Can you work these out from the model? Positions are in its coordinate system, mm. Coordinates: 2 decimals unless noted, no trailing zeros. Order: outer loops, then holes, each group sorted by start corner. A loop starts at its lowest first (then second) coordinate and runs counter-clockwise, first axis right, second up.
Autodesk Inventor part; units mm, degrees
ref_plane "Start Plane" through (0, 0, -57.0711) normal (0, 0, 1) x (1, 0, 0)
ref_plane "End Plane" through (0, 0, 2457.0711) normal (0, 0, 1) x (1, 0, 0)
ref_plane "Work Plane4" through (-60, 0, 2460) normal (0.7071, 0, 0.7071) x (0.7071, 0, -0.7071)
ref_plane "Start Plane" through (0, 0, -57.0711) normal (0, 0, 1) x (1, 0, 0)
ref_plane "End Plane" through (0, 0, 2457.0711) normal (0, 0, 1) x (1, 0, 0)
sketch "Sketch" plane through (0, 0, 0) normal (0, 0, 1) x (1, 0, 0)
  line L0 (-60, -50) -> (-60, 50)
  line L1 (-50, 60) -> (50, 60)
  line L2 (60, 50) -> (60, -50)
  line L3 (50, -60) -> (-50, -60)
  arc A0 (-60, -50) -> (-50, -60) centre (-50, -50) ccw
  arc A1 (60, 50) -> (50, 60) centre (50, 50) ccw
  arc A2 (-50, 60) -> (-60, 50) centre (-50, 50) ccw
  arc A3 (50, -60) -> (60, -50) centre (50, -50) ccw
  arc A4 (-50, 55) -> (-55, 50) centre (-50, 50) ccw
  line L4 (-50, 55) -> (50, 55)
  arc A5 (55, 50) -> (50, 55) centre (50, 50) ccw
  line L5 (55, 50) -> (55, -50)
  arc A6 (50, -55) -> (55, -50) centre (50, -50) ccw
  line L6 (50, -55) -> (-50, -55)
  arc A7 (-55, -50) -> (-50, -55) centre (-50, -50) ccw
  line L7 (-55, -50) -> (-55, 50)
  line L8 (0, 86.8995) -> (0, -86.8995) construction
  line L9 (-86.8995, 0) -> (86.8995, 0) construction
  dimension "d7" = 10
  dimension "d9" = 120
  dimension "d11" = 120
  dimension "d12" = 5
  dimension "d15" = 60
  dimension "d16" = 60
extrude "Body" add sketch "Sketch" along normal up to surface (2514.1421 mm away) from surface at -57.0711
sketch "Sketch3" plane through (0, 0, 0) normal (0, 0, 1) x (1, 0, 0)
  line L0 (0, 0) -> (10, 0)
ref_plane "Work Plane3" through (0, 0, 0) normal (0, -1, 0) x (1, 0, 0)
ref_plane "Work Plane4" through (-60, 0, 2460) normal (0.7071, 0, 0.7071) x (0.7071, 0, -0.7071)
split "Split1" plane through (-60, 0, 2460) removes the side toward (0.7071, 0, 0.7071)
ref_plane "Work Plane5" through (0, -60, 2460) normal (0, 0.7071, 0.7071) x (1, 0, 0)
split "Split2" plane through (0, -60, 2460) removes the side toward (0, 0.7071, 0.7071)
ref_plane "Work Plane6" through (0, -60, -60) normal (0, 0.7071, -0.7071) x (1, 0, 0)
split "Split3" plane through (0, -60, -60) removes the side toward (0, 0.7071, -0.7071)
ref_plane "Work Plane7" through (-60, 0, -60) normal (0.7071, 0, -0.7071) x (-0.7071, 0, -0.7071)
split "Split4" plane through (-60, 0, -60) removes the side toward (0.7071, 0, -0.7071)
sketch "Sketch4" plane through (0, 0, 0) normal (0, -1, 0) x (1, 0, 0)
  line L0 (-2, -57.0711) -> (12, -57.0711)
  line L1 (-2, 2457.0711) -> (12, 2457.0711)
  dimension "d18" = 2514.1421
equation "\"d7\" = G_IR"
equation "\"d9\" = G_W"
equation "\"d11\" = G_H"
equation "\"d12\" = G_T"
equation "\"d15\" = 0.5 * d9"
equation "\"d16\" = 0.5 * d11"
equation "\"d3\" = G_L"
equation "\"G_W\" = 120"
equation "\"G_H\" = 120"
equation "\"G_T\" = 5"
equation "\"G_IR\" = 10"
equation "\"G_L\" = d18"
equation "\"G_OFFSET_START\" = 57.07107"
equation "\"G_OFFSET_END\" = 57.07107"
equation "\"d13\" = -G_OFFSET_START"
equation "\"d14\" = G_OFFSET_END + B_L"
properties part number "ISO 10799-2 - 120x120x5 - 2514,14" material "Steel, Mild"
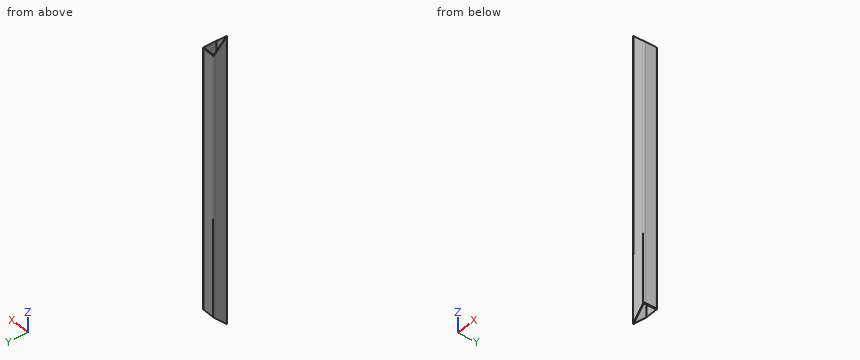
1. Please list where these lines run through material, in increasing order: probe 1 along X at (y, z) = (37.5, 500.5); probe 2 along X at (y, z) = (23, 2352.5).
Completed:
probe 1: x = -60 to -55, 55 to 60
probe 2: x = -60 to -55
2. Imagine slicing it at B-B on y = -6.5. Please give me the cut outline in (x, z).
Completed:
outline: (-60, -6.5) - (-55, -6.5) - (-55, 2406.5) - (-60, 2406.5) - close; (55, 55) - (60, 60) - (60, 2340) - (55, 2345) - close
3. Imagine slicing it at A-A on x = 13.5. Please give me the cut outline in (y, z).
Completed:
outline: (-60, 13.5) - (-55, 13.5) - (-55, 2386.5) - (-60, 2386.5) - close; (55, 55) - (60, 60) - (60, 2340) - (55, 2345) - close
4. Imagine slicing it at C-C on z = 351.5. Please give me the cut outline in (x, y).
Completed:
outline: (-60, -50) arc R10 ccw to (-50, -60) - (50, -60) arc R10 ccw to (60, -50) - (60, 50) arc R10 ccw to (50, 60) - (-50, 60) arc R10 ccw to (-60, 50) - close; hole (-55, -50) arc R5 ccw to (-50, -55) - (50, -55) arc R5 ccw to (55, -50) - (55, 50) arc R5 ccw to (50, 55) - (-50, 55) arc R5 ccw to (-55, 50) - close
